```python
from build123d import *

# Parameters (mm, degrees)
BOSS_EXTRUDE1_DEPTH = 200
CUT_EXTRUDE1_DEPTH  = 30
CUT_EXTRUDE2_DEPTH  = 75.627789266
CUT_EXTRUDE3_DEPTH  = 75.627789266
SKETCH5_R           = 50
BOSS_EXTRUDE2_DEPTH = 30


with BuildPart() as part:
    # Sketch1 → Boss-Extrude1 (new body)
    with BuildSketch(Plane(origin=(0, 0, 0), x_dir=(1, 0, 0), z_dir=(0, 1, 0))):
        Polygon((-250, 0), (250, 0), (250, 25), (100, 40), (100, 50), (-100, 50), (-100, 40), (-250, 25), align=None)
    extrude(amount=BOSS_EXTRUDE1_DEPTH)

    # Sketch2 → Cut-Extrude1 (cut)
    with BuildSketch(Plane(origin=(0, 0, -50), x_dir=(-1, 0, 0), z_dir=(0, 0, -1))):
        with BuildLine():
            Line((-40, 0), (40, 0))
            Line((40, 0), (40, 90.399951474))
            ThreePointArc((40, 90.399951474), (0, 130.399951474), (-40, 90.399951474))
            Line((-40, 90.399951474), (-40, 0))
        make_face()
    extrude(amount=-CUT_EXTRUDE1_DEPTH, mode=Mode.SUBTRACT)

    # Sketch3 → Cut-Extrude2 (cut, through all)
    with BuildSketch(Plane(origin=(-4.95049505, 0, -49.504950495), x_dir=(-0.99503719, 0, 0.099503719), z_dir=(-0.099503719, 0, -0.99503719))):
        with BuildLine():
            Line((186.271704577, 130), (296.385375979, 130))
            Line((296.385375979, 130), (296.385375979, 70))
            Line((296.385375979, 70), (186.271704577, 70))
            ThreePointArc((186.271704577, 70), (156.271704577, 100), (186.271704577, 130))
        make_face()
    extrude(amount=-CUT_EXTRUDE2_DEPTH, mode=Mode.SUBTRACT)

    # Sketch4 → Cut-Extrude3 (cut, through all)
    with BuildSketch(Plane(origin=(4.95049505, 0, -49.504950495), x_dir=(-0.99503719, 0, -0.099503719), z_dir=(0.099503719, 0, -0.99503719))):
        with BuildLine():
            Line((-186.271704577, 130), (-315.600266526, 130))
            Line((-315.600266526, 130), (-315.600266526, 70))
            Line((-315.600266526, 70), (-186.271704577, 70))
            ThreePointArc((-186.271704577, 70), (-156.271704577, 100), (-186.271704577, 130))
        make_face()
    extrude(amount=-CUT_EXTRUDE3_DEPTH, mode=Mode.SUBTRACT)

    # Sketch5 → Boss-Extrude2 (add)
    with BuildSketch(Plane(origin=(0, 200, 0), x_dir=(1, 0, 0), z_dir=(0, 1, 0))):
        with BuildLine():
            Line((100, 50), (-100, 50))
            Line((-100, 50), (-100, 176.90746365))
            ThreePointArc((-100, 176.90746365), (0, 276.90746365), (100, 176.90746365))
            Line((100, 176.90746365), (100, 50))
        make_face()
        with Locations((0, 176.90746365)):
            Circle(SKETCH5_R, mode=Mode.SUBTRACT)
    extrude(amount=-BOSS_EXTRUDE2_DEPTH)


solid = part.part
```
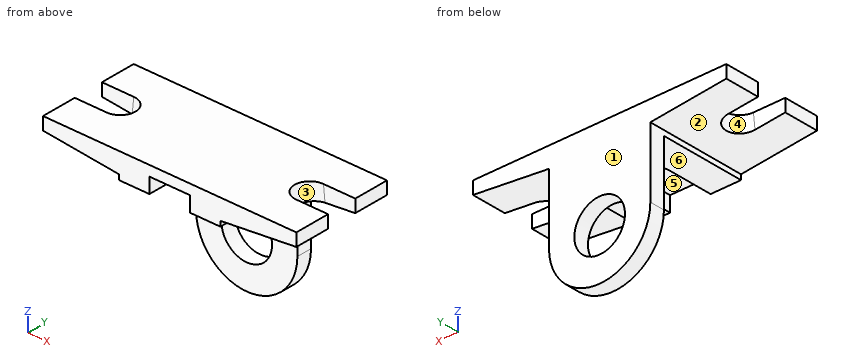
Input: part model. Units: mm. Frame: model coordinates. Face numbers are marked on the shaded views. A direction names the side the tool comes from. Round coordinates to 2 decimals unless told otherwise and drop trailing zeros. Order: outer loops, then holes, each group sorted by start corner. A loop starts at its lowest first (then second) coordinate and runs counter-clockwise, first axis right, second up. Notation, with made-up numbers: (51, 20.25) - (83, 20.25) arc R26 ccw to (83, 43.25) - close; hole circle Ø9 at (13.25, 12.25). An arc over 180 degrees is marked (long way). Answer in a Markdown table with one row per item.
Item 1: Reachability of the marked faces 4, 5 and 6 from +Z, -Z, +X, -X, +Y, -Y: full face, straight path, thin tool, end or side. Return the list, or none.
Model answer:
| item | result |
|---|---|
| face 4 | +Z, -X |
| face 5 | -Z, -Y |
| face 6 | -Z, +X, -X, -Y |
Item 2: Mould query, pull axis Y, two halves, no side actions, for the marked faces 1, 2 and 3. Classes: released by +Y, released by -Y, zero draft, split by the parting line, or undercut.
Model answer:
| item | result |
|---|---|
| face 1 | released by +Y |
| face 2 | zero draft |
| face 3 | undercut |
Item 3: Pin query (flat end, axial travel): pin 1 (3 mm diameter, centred on x = -19.5, z = -128.5, fed in from -Y); pin 2 (1.5 mm diameter, centred on x = -109, y = 164.5, fed in from -Z) (3 decimals). Return the tip coordinate at first contact, or that it passes through.
Model answer:
| item | result |
|---|---|
| pin 1 | stops at y = 170 |
| pin 2 | stops at z = -39.175 |
Item 4: Section query C-C (y = 159). Return the cut outline in (x, z), then the cut area to 4 significant figures.
Model answer:
| item | result |
|---|---|
| outline | (-250, -25) - (-100, -40) - (-100, -50) - (100, -50) - (100, -40) - (250, -25) - (250, 0) - (-250, 0) - close |
| area | 19,750 mm² |
Item 5: Line query: line 1 (X direction, y = 88.5, z = -41.5); line 2 (Z direction, x = 0, y = 192); line 3 (Y direction, x = -91.5, z = -166.5). Output: solid intervals per line, ascending.
Model answer:
| item | result |
|---|---|
| line 1 | x = -100 to -40, 40 to 100 |
| line 2 | z = -276.91 to -226.91, -126.91 to 0 |
| line 3 | y = 170 to 200 |
Item 6: Section query A-A (x = 204). Return the cut outline in (y, z), then the cut area to 3 significant figures.
Model answer:
| item | result |
|---|---|
| outline | (0, -29.6) - (70, -29.6) - (70, 0) - (0, 0) - close; (130, -29.6) - (200, -29.6) - (200, 0) - (130, 0) - close |
| area | 4,140 mm² |
Item 7: Section query B-B (z = -168). Return the cut outline in (x, y), then the cut area to 3 significant figures.
Model answer:
| item | result |
|---|---|
| outline | (-100, 170) - (-49.2, 170) - (-49.2, 200) - (-100, 200) - close; (49.2, 170) - (100, 170) - (100, 200) - (49.2, 200) - close |
| area | 3,050 mm² |
Item 8: Section query D-D (x = 0). Return the cut outline in (y, z).
Model answer:
| item | result |
|---|---|
| outline | (0, -20) - (130.4, -20) - (130.4, -50) - (170, -50) - (170, -126.91) - (200, -126.91) - (200, 0) - (0, 0) - close; (170, -276.91) - (200, -276.91) - (200, -226.91) - (170, -226.91) - close |
